Work out the finished part from the listing and answer in its coordinate system (mm). A direction names the side the tool comes from. Coordinates: 2 decimals unless noted, no trailing zeros. Order: outer loops, then holes, each group sorted by start corner. A loop starts at its lowest first (then second) coordinate and runs counter-clockwise, first axis right, second up. Notation, with made-up numbers: M 17,21 L 56,21 A22 cw 56,41 Z; hole C 73,5 d2. An arc over 180 degrees is marked long. Use a Markdown table: item, result.
from build123d import *

# Parameters (mm, degrees)
SKETCH1_W               = 40
SKETCH1_H               = 40
BOSS_EXTRUDE1_DEPTH     = 3
SKETCH2_W               = 40
SKETCH2_H               = 6
BOSS_EXTRUDE2_DEPTH     = 3
SKETCH4_W               = 43
SKETCH4_H               = 6
BOSS_EXTRUDE3_DEPTH     = 3
SKETCH5_W               = 43
SKETCH5_H               = 6
BOSS_EXTRUDE4_DEPTH     = 3
SKETCH6_W               = 46
SKETCH6_H               = 6
BOSS_EXTRUDE5_DEPTH     = 3
SKETCH7_W               = 30
SKETCH7_H               = 2
CUT_EXTRUDE1_DEPTH      = 3
MIRROR2_COPY_1_SKETCH_W = 30
MIRROR2_COPY_1_SKETCH_H = 2
MIRROR2_COPY_1_DEPTH    = 3
SKETCH8_W               = 10
SKETCH8_H               = 10
SKETCH8_W_2             = 7.999655552
SKETCH8_H_2             = 7.999655552
BOSS_EXTRUDE6_DEPTH     = 3
SKETCH9_R               = 0.8
CUT_EXTRUDE2_DEPTH      = 3
SKETCH10_R              = 0.5
CUT_EXTRUDE3_DEPTH      = 10


with BuildPart() as part:
    # Sketch1 → Boss-Extrude1 (new body)
    with BuildSketch(Plane(origin=(0, 0, 0), x_dir=(1, 0, 0), z_dir=(0, 1, 0))):
        with Locations((-20, -20)):
            Rectangle(SKETCH1_W, SKETCH1_H)
    extrude(amount=BOSS_EXTRUDE1_DEPTH)



with BuildPart() as body_2:
    # Sketch2 → Boss-Extrude2 (new body)
    with BuildSketch(Plane(origin=(0, 0, 0), x_dir=(0, 0, -1), z_dir=(1, 0, 0))):
        with Locations((-20, 3)):
            Rectangle(SKETCH2_W, SKETCH2_H)
    extrude(amount=BOSS_EXTRUDE2_DEPTH)


with BuildPart() as part_1:
    add(part.part)

    add(body_2.part)  # Boss-Extrude3 merges body 2
    # Sketch4 → Boss-Extrude3 (add)
    with BuildSketch(Plane.XY.offset(40)):
        with Locations((-18.5, 3)):
            Rectangle(SKETCH4_W, SKETCH4_H)
    extrude(amount=BOSS_EXTRUDE3_DEPTH)

    # Sketch5 → Boss-Extrude4 (add)
    with BuildSketch(Plane(origin=(0, 0, 0), x_dir=(-1, 0, 0), z_dir=(0, 0, -1))):
        with Locations((18.5, 3)):
            Rectangle(SKETCH5_W, SKETCH5_H)
    extrude(amount=BOSS_EXTRUDE4_DEPTH)

    # Sketch6 → Boss-Extrude5 (add)
    with BuildSketch(Plane.ZY.offset(40)):
        with Locations((20, 3)):
            Rectangle(SKETCH6_W, SKETCH6_H)
    extrude(amount=BOSS_EXTRUDE5_DEPTH)

    # Sketch7 → Cut-Extrude1 (cut)
    with BuildSketch(Plane.ZY):
        with Locations((20, 4.5)):
            Rectangle(SKETCH7_W, SKETCH7_H)
    cut_extrude1 = extrude(amount=-CUT_EXTRUDE1_DEPTH, mode=Mode.SUBTRACT)

    # Mirror1: Cut-Extrude1 across plane
    add(cut_extrude1.mirror(Plane(origin=(0, 0, 0), x_dir=(-0.707106781, 0, 0.707106781), z_dir=(0.707106781, 0, 0.707106781))), mode=Mode.SUBTRACT)

    # Mirror2: Cut-Extrude1 across plane
    add(cut_extrude1.mirror(Plane(origin=(-20, 0, 20), x_dir=(0.707106781, 0, 0.707106781), z_dir=(0.707106781, 0, -0.707106781))), mode=Mode.SUBTRACT)

    # Mirror2 copy 1 sketch → Mirror2 copy 1 (cut)
    with BuildSketch(Plane(origin=(-40, 0, 40), x_dir=(0, 0, -1), z_dir=(1, 0, 0))):
        with Locations((20, 4.5)):
            Rectangle(MIRROR2_COPY_1_SKETCH_W, MIRROR2_COPY_1_SKETCH_H)
    extrude(amount=-MIRROR2_COPY_1_DEPTH, mode=Mode.SUBTRACT)

    # Sketch8 → Boss-Extrude6 (add)
    with BuildSketch(Plane(origin=(0, 3, 0), x_dir=(1, 0, 0), z_dir=(0, 1, 0))):
        with Locations((-20, -20)):
            Rectangle(SKETCH8_W, SKETCH8_H)
        with Locations((-20, -20)):
            Rectangle(SKETCH8_W_2, SKETCH8_H_2, mode=Mode.SUBTRACT)
    extrude(amount=BOSS_EXTRUDE6_DEPTH)

    # Sketch9 → Cut-Extrude2 (cut)
    with BuildSketch(Plane(origin=(0, 3, 0), x_dir=(1, 0, 0), z_dir=(0, 1, 0))):
        with Locations((-20, -20)):
            Circle(SKETCH9_R)
    extrude(amount=-CUT_EXTRUDE2_DEPTH, mode=Mode.SUBTRACT)

    # Sketch10 → Cut-Extrude3 (cut)
    with BuildSketch(Plane.ZY.offset(25)):
        with Locations((20, 4.5)):
            Circle(SKETCH10_R)
    cut_extrude3 = extrude(amount=-CUT_EXTRUDE3_DEPTH, mode=Mode.SUBTRACT)

    # Mirror3: Cut-Extrude3 across plane
    add(cut_extrude3.mirror(Plane(origin=(-20, 0, 20), x_dir=(0.707106781, 0, 0.707106781), z_dir=(0.707106781, 0, -0.707106781))), mode=Mode.SUBTRACT)


solid = part_1.part
1. Find the intervals of material crossed by probe 1 along Z at (x, y) = (-18, 3.35); probe 2 along X at (y, z) = (4.5, 24.3); probe 3 along Z at (x, y) = (-20.5, 3.6), in increasing order.
Answers below:
| item | result |
|---|---|
| probe 1 | -3 to 0, 15 to 16, 24 to 25, 40 to 43 |
| probe 2 | -25 to -20.5, -19.5 to -15 |
| probe 3 | 15 to 16, 24 to 25 |
2. For faces 1 (the face through (1, 3.5, 20)), 2 (the face through (-20, 3.5, -1)), 3 (the face through (-20, 5.5, 41)), 4 (the face through (1, 4, 5)), 5 (the face through (-20.07, 5.15, 15)), determine the directions among +Z, -Z, +X, -X, +Y, -Y from which every point of the face is accessible in a straight line to the end or side of a thin tool.
Answers below:
| item | result |
|---|---|
| face 1 | +X |
| face 2 | -Z |
| face 3 | +Z |
| face 4 | +X, -X |
| face 5 | +Y |
3. For a pull along X with two mould halves and no side action, classify faces 6 (the face through (-41, 4, 35)), 7 (the face through (-20, 5.5, -1)), 8 (the face through (-25, 5.15, 20.07)) as +X half, -X half, draft (parallel to the pull), parting line (faces both ways), or undercut.
Answers below:
| item | result |
|---|---|
| face 6 | draft |
| face 7 | undercut |
| face 8 | undercut |
4. Section B-B on x = -17 is taken. Determine the outline of the cut face in (y, z).
Answers below:
| item | result |
|---|---|
| outline | M 0,-3 L 3.5,-3 L 3.5,0 L 3,0 L 3,15 L 6,15 L 6,16 L 3,16 L 3,24 L 6,24 L 6,25 L 3,25 L 3,40 L 3.5,40 L 3.5,43 L 0,43 Z; M 5.5,-3 L 6,-3 L 6,0 L 5.5,0 Z; M 5.5,40 L 6,40 L 6,43 L 5.5,43 Z |
5. Section D-D on x = -28.5 is taken. Determine the outline of the cut face in (y, z), then the cut area to 3 significant figures.
Answers below:
| item | result |
|---|---|
| outline | M 0,-3 L 3.5,-3 L 3.5,0 L 3,0 L 3,40 L 3.5,40 L 3.5,43 L 0,43 Z; M 5.5,-3 L 6,-3 L 6,0 L 5.5,0 Z; M 5.5,40 L 6,40 L 6,43 L 5.5,43 Z |
| area | 144 mm² |
6. Section C-C on x = -3.5 is taken. Determine the outline of the cut face in (y, z).
Answers below:
| item | result |
|---|---|
| outline | M 0,-3 L 6,-3 L 6,0 L 3,0 L 3,40 L 6,40 L 6,43 L 0,43 Z |
7. Section A-A on z = 28 is taken. Determine the outline of the cut face in (x, y).
Answers below:
| item | result |
|---|---|
| outline | M -43,0 L 3,0 L 3,3.5 L 0,3.5 L 0,3 L -40,3 L -40,3.5 L -43,3.5 Z; M -43,5.5 L -40,5.5 L -40,6 L -43,6 Z; M 0,5.5 L 3,5.5 L 3,6 L 0,6 Z |
8. Flat-ended cylindrical pins translate along their axes: P1, Ø3, axis at y = 5, z = 20, coming from the -X side; P2, Ø0.9, axis at x = -22, y = 4.5, coming from the +Z side; P3, Ø1.5, axis at x = -12.5, z = 20.5, coming from the +Y side; P4, Ø0.9, axis at x = -18.5, y = 5, coming from the -Z side. Find the tip coordinate at first contact, or state that the pin passes through.
Answers below:
| item | result |
|---|---|
| P1 | x = -43 |
| P2 | z = 25 |
| P3 | y = 3 |
| P4 | z = 15 |
